Verification items for the finished model (mm, model axes). A direction names the side the tool comes from. Round coordinates to 2 decimals unless told otherwise and drop trailing zeros. Write each loop counter-clockwise with the first axis right and the second up, starting at its lowest first coordinate (ties: lowest second). Pieces come first, ordered by that corner, then holes. Notation, with made-up numbers: (14.25, 34) - (22.25, 34) arc R27 ccw to (22.25, 51) - close; hole circle Ø6 at (14, 87). An arc over 180 degrees is marked (long way). Answer as a JSON object with one key per item and string values. Group by question number.
1) Set-up check for faces 1 (the flat face through (56, -6, 66)), 2 (the cylindrical face through (8.04, -2.96, 71.23)), 3 (the cylindrical face through (56.96, -9.04, 81.23)): record each of +Z, -Z, +X, -X, +Y, -Y from which the full face is reachable in a straight line by a thin tool's end or side.
2) Thickness scan on line 1 (X direction, y = -10.55, z = 45); line 2 (Z direction, x = 25.5, y = -8.25); line 3 (Z direction, x = 10, y = -7.9). Record the ranges inside material, lowest first.
3) Section check A-A (z = 20). Enter the section's corners in (x, y).
4) Section check D-D (y = -10.75). Enter the section's corners in (x, z).
5) Section check C-C (z = 75). Enter the section's corners in (x, y), then the cut area to 3 significant figures.
6) Go/stop test with flat-tipped pins: pin 1 Ø3.5 at (x, z) = (10, 45) entering from -Y; pin 2 Ø6 at (x, y) = (55, -8.5) entering from -Z; pin 3 Ø7 at (x, z) = (10.5, 45) entering from +Y. Record where each tip stops, or that it passes through.
7) Mould release check, pull along X, two halves, no side actions. Record for faces 4 (the flat face through (50, -6, 42)), 5 (the cylindrical face through (9.642, -8.958, 77.727)), 6 (the flat face through (0, -6, 39)), 7 (the cylindrical face through (37.973, -8.958, 46.859)): +X half, -X half, draft (parallel to the pull), parting line (faces both ways), or undercut.
8) Section check B-B (x = 40). Enter the section's corners in (y, z).
```python
from build123d import *

# Parameters (mm, degrees)
F0_R     = 2.75
F0_R_2   = 13.25
F1_DEPTH = 12
F2_R     = 4.25
F3_DEPTH = 6
F4_R     = 4.25
F5_DEPTH = 6


with BuildPart() as f1:
    # F0 (on Front) → F1 (new body)
    with BuildSketch(Plane.XZ):
        Polygon((19, 93), (0, 77), (0, 0), (30, 0), (50, 19), (50, 66), (63, 66), (63, 93), align=None)
        with Locations((25, 20)):
            Circle(F0_R, mode=Mode.SUBTRACT)
        with Locations((10, 45)):
            Circle(F0_R, mode=Mode.SUBTRACT)
        with Locations((40, 45)):
            Circle(F0_R, mode=Mode.SUBTRACT)
        with Locations((25, 60)):
            Circle(F0_R_2, mode=Mode.SUBTRACT)
        with Locations((10, 75)):
            Circle(F0_R, mode=Mode.SUBTRACT)
        with Locations((40, 75)):
            Circle(F0_R, mode=Mode.SUBTRACT)
        with Locations((55, 85)):
            Circle(F0_R, mode=Mode.SUBTRACT)
    extrude(amount=F1_DEPTH)

    # F2 (on face) → F3 (cut)
    with BuildSketch(Plane.XZ.offset(12)):
        with Locations((55, 85)):
            Circle(F2_R)
        with Locations((25, 20)):
            Circle(F2_R)
    extrude(amount=-F3_DEPTH, mode=Mode.SUBTRACT)

    # F4 (on face) → F5 (cut)
    with BuildSketch(Plane(origin=(0, 0, 0), x_dir=(-1, 0, 0), z_dir=(0, 1, 0))):
        with Locations((-10, 75)):
            Circle(F4_R)
        with Locations((-40, 75)):
            Circle(F4_R)
        with Locations((-40, 45)):
            Circle(F4_R)
        with Locations((-10, 45)):
            Circle(F4_R)
    extrude(amount=-F5_DEPTH, mode=Mode.SUBTRACT)


solid = f1.part
```
Returned:
{
 "1": {"face 1": "-Z, +X, +Y, -Y", "face 2": "+Y", "face 3": "-Y"},
 "2": {"line 1": "0 to 7.25, 12.75 to 37.25, 42.75 to 50", "line 2": "0 to 15.78, 24.22 to 46.76, 73.24 to 93", "line 3": "0 to 42.25, 47.75 to 72.25, 77.75 to 85.42"},
 "3": {"outline": "(0, -12) - (20.75, -12) - (20.75, -6) - (22.25, -6) - (22.25, 0) - (0, 0) - close; (27.75, -6) - (29.25, -6) - (29.25, -12) - (50, -12) - (50, 0) - (27.75, 0) - close"},
 "4": {"outline": "(0, 0) - (30, 0) - (50, 19) - (50, 66) - (63, 66) - (63, 93) - (19, 93) - (0, 77) - close; hole circle Ø5.5 at (10, 45); hole circle Ø5.5 at (10, 75); hole circle Ø26.5 at (25, 60); hole circle Ø8.5 at (25, 20); hole circle Ø5.5 at (40, 45); hole circle Ø5.5 at (40, 75); hole circle Ø8.5 at (55, 85)"},
 "5": {"outline": "(0, -12) - (7.25, -12) - (7.25, -6) - (5.75, -6) - (5.75, 0) - (0, 0) - close; (12.75, -12) - (37.25, -12) - (37.25, -6) - (35.75, -6) - (35.75, 0) - (14.25, 0) - (14.25, -6) - (12.75, -6) - close; (42.75, -12) - (63, -12) - (63, 0) - (44.25, 0) - (44.25, -6) - (42.75, -6) - close", "area": "588 mm2"},
 "6": {"pin 1": "through", "pin 2": "z = 66", "pin 3": "y = -6"},
 "7": {"face 4": "+X half", "face 5": "undercut", "face 6": "-X half", "face 7": "undercut"},
 "8": {"outline": "(-12, 9.5) - (0, 9.5) - (0, 40.75) - (-6, 40.75) - (-6, 42.25) - (-12, 42.25) - close; (-12, 47.75) - (-6, 47.75) - (-6, 49.25) - (0, 49.25) - (0, 70.75) - (-6, 70.75) - (-6, 72.25) - (-12, 72.25) - close; (-12, 77.75) - (-6, 77.75) - (-6, 79.25) - (0, 79.25) - (0, 93) - (-12, 93) - close"}
}
